Verification items for the finished model (mm, model axes). A direction names the side the tool comes from. Coordinates: 2 decimals unless noted, no trailing zeros. Order: outer loops, then holes, each group sorted by start corner. A loop starts at its lowest first (then second) coordinate and runs counter-clockwise, first axis right, second up. Notation, with made-up numbers: M 15.5,38 L 46.5,38 A27 ccw 46.5,70 Z; hole C -16,70.25 d7. An arc over 180 degrees is marked long. Return JSON: item names as keys, results as strings. Group by question number.
Q1. Thickness scan on probe 1 along X at (y, z) = (-2.75, 1); probe 2 along X at (y, z) = (6.75, 12); probe 3 along Y at (x, z) = (6.5, 3.5). Record the ranges inside material, lowest first.
Q2. Go/stop test with flat-tipped pins: pin 1 Ø3.5 at (x, z) = (5.64, -18.02) entering from +Y; pin 2 Ø1.8 at (x, y) = (0.64, 13) entering from +Z; pin 3 Ø6.5 at (x, z) = (0, -11.5) entering from -Y; pin 4 Ø6 at (x, z) = (5.5, 5.5) entering from +Y. Record where each tip stops, or that it passes through.
Q3. Section check C-C, the plane z = -17. Enter the section's corners in (x, y).
Q4. Section check A-A, the plane y = -4.25. Enter the section's corners in (x, z).
Q5. Section check B-B, the plane x = 0.75. Enter the section's corners in (y, z).
Q6. Section check D-D, the plane y = 3. Enter the section's corners in (x, z).
Q7. Access from +Z, -Z, +X, -X, +Y, -Y to the whole of each face (thin tool, end or side, straight path). Record for faces 5 (the face through (0, -3, 7)), 6 (the face through (0.318, 11.536, 16.512)), 7 (the face through (1, 8, 13.977)), 8 (the face through (-4, -1, -20.873)), 9 (the face through (-4.682, -3.972, -19.487)).
Q8. Mould release check, pull along Z, two halves, no side actions. Record for faces 1 (the face through (1, 0, -3)), 2 (the face through (-5.547, -3.972, 0.064)), 3 (the face through (-5.385, 8.112, 9.047)), 4 (the face through (7.976, -0.986, -16.363)): pulls with the +Z half, pulls with the -Z half, needs draft (parallel to the pull), parting line crosses it, or undercut.
from build123d import *

# Parameters (mm, degrees)
F0_W      = 16
F0_H      = 40
F0_R      = 1.5
F0_W_2    = 8
F0_H_2    = 14
F0_W_3    = 10
F0_H_3    = 4.5
F1_DEPTH  = 6
F2_DEPTH  = 3
F3_W      = 16
F3_H      = 16
F3_R      = 1.5
F4_DEPTH  = 5
F7_DEPTH  = 2
F9_DEPTH  = 4
F10_START = -12
F10_DEPTH = 4


with BuildPart() as f1:
    # F0 (on Front) → F1 (new body)
    with BuildSketch(Plane.XZ):
        with Locations((0.6433322058, -1.0231063997)):
            Rectangle(F0_W, F0_H)
        with Locations((-4.3566677942, -18.0231063997)):
            Circle(F0_R, mode=Mode.SUBTRACT)
        with Locations((0.6433322058, -8.5231063997)):
            Rectangle(F0_W_2, F0_H_2, mode=Mode.SUBTRACT)
        with Locations((5.6433322058, -18.0231063997)):
            Circle(F0_R, mode=Mode.SUBTRACT)
        with Locations((-4.3566677942, 0.9768936003)):
            Circle(F0_R, mode=Mode.SUBTRACT)
        with Locations((0.246625971, 7.2268936003)):
            Rectangle(F0_W_3, F0_H_3, mode=Mode.SUBTRACT)
        with Locations((5.6433322058, 0.9768936003)):
            Circle(F0_R, mode=Mode.SUBTRACT)
    extrude(amount=F1_DEPTH)

    # F0 (on Front) → F2 (join)
    with BuildSketch(Plane.XZ):
        with Locations((0.246625971, 7.2268936003)):
            Rectangle(F0_W_3, F0_H_3)
        with Locations((0.6433322058, -8.5231063997)):
            Rectangle(F0_W_2, F0_H_2)
    extrude(amount=F2_DEPTH)

    # F3 (on face) → F4 (join)
    with BuildSketch(Plane.XY.offset(18.9768936003)):
        with Locations((0.6433322058, 8)):
            Rectangle(F3_W, F3_H)
        with Locations((0.6433322058, 3)):
            Circle(F3_R, mode=Mode.SUBTRACT)
        with Locations((0.6433322058, 13)):
            Circle(F3_R, mode=Mode.SUBTRACT)
    extrude(amount=-F4_DEPTH)

    # F6 (on face) → F7 (cut)
    with BuildSketch(Plane.XZ):
        Polygon((7.288780473, 3.8268936003), (3.9978839386, 3.8268936003), (2.3524356714, 0.9768936003), (3.9978839386, -1.8731063997), (7.288780473, -1.8731063997), (8.9342287402, 0.9768936003), align=None)
        Polygon((-2.711219527, 3.8268936003), (-6.0021160614, 3.8268936003), (-7.6475643286, 0.9768936003), (-6.0021160614, -1.8731063997), (-2.711219527, -1.8731063997), (-1.0657712598, 0.9768936003), align=None)
        Polygon((-2.711219527, -15.1731063997), (-6.0021160614, -15.1731063997), (-7.6475643286, -18.0231063997), (-6.0021160614, -20.8731063997), (-2.711219527, -20.8731063997), (-1.0657712598, -18.0231063997), align=None)
        Polygon((7.288780473, -15.1731063997), (3.9978839386, -15.1731063997), (2.3524356714, -18.0231063997), (3.9978839386, -20.8731063997), (7.288780473, -20.8731063997), (8.9342287402, -18.0231063997), align=None)
    extrude(amount=F7_DEPTH, mode=Mode.SUBTRACT)

    # F8 (on face) → F9 (join)
    with BuildSketch(Plane(origin=(-7.3566677942, 0, 0), x_dir=(0, -1, 0), z_dir=(-1, 0, 0))):
        Polygon((-16, 13.9768936003), (0, 3.9768936003), (0, 13.9768936003), align=None)
    extrude(amount=-F9_DEPTH)

    # F8 (on face) → F10 (join)
    with BuildSketch(Plane(origin=(-7.3566677942, 0, 0), x_dir=(0, -1, 0), z_dir=(-1, 0, 0)).offset(F10_START)):
        Polygon((-16, 13.9768936003), (0, 3.9768936003), (0, 13.9768936003), align=None)
    extrude(amount=-F10_DEPTH)


solid = f1.part
Numbers:
{
 "1": {"probe 1": "x = -7.36 to -5.86, -2.86 to 4.14, 7.14 to 8.64", "probe 2": "x = -7.36 to -3.36, 4.64 to 8.64", "probe 3": "y = -6 to -2"},
 "2": {"pin 1": "stops at y = -2", "pin 2": "passes through", "pin 3": "stops at y = -3", "pin 4": "stops at y = 7.24"},
 "3": {"outline": "M -7.36,-6 L -5.45,-6 L -5.45,-2 L -7.06,-2 L -7.06,0 L -7.36,0 Z; M -3.26,-6 L 4.55,-6 L 4.55,-2 L 2.94,-2 L 2.94,0 L -1.66,0 L -1.66,-2 L -3.26,-2 Z; M 6.74,-6 L 8.64,-6 L 8.64,0 L 8.34,0 L 8.34,-2 L 6.74,-2 Z"},
 "4": {"outline": "M -7.36,-21.02 L 8.64,-21.02 L 8.64,18.98 L -7.36,18.98 Z; hole C -4.36,-18.02 d3; hole C -4.36,0.98 d3; hole M -4.75,4.98 L 5.25,4.98 L 5.25,9.48 L -4.75,9.48 Z; hole M -3.36,-15.52 L 4.64,-15.52 L 4.64,-1.52 L -3.36,-1.52 Z; hole C 5.64,-18.02 d3; hole C 5.64,0.98 d3"},
 "5": {"outline": "M -6,-21.02 L 0,-21.02 L 0,13.98 L 1.5,13.98 L 1.5,18.98 L -6,18.98 L -6,9.48 L -3,9.48 L -3,4.98 L -6,4.98 L -6,-1.52 L -3,-1.52 L -3,-15.52 L -6,-15.52 Z; M 4.5,13.98 L 11.5,13.98 L 11.5,18.98 L 4.5,18.98 Z; M 14.5,13.98 L 16,13.98 L 16,18.98 L 14.5,18.98 Z"},
 "6": {"outline": "M -7.36,5.85 L -3.36,5.85 L -3.36,13.98 L -0.86,13.98 L -0.86,18.98 L -7.36,18.98 Z; M 2.14,13.98 L 4.64,13.98 L 4.64,5.85 L 8.64,5.85 L 8.64,18.98 L 2.14,18.98 Z"},
 "7": {"face 5": "-Y", "face 6": "+Z, -Z", "face 7": "-Z, +Y", "face 8": "+Y", "face 9": "+Y, -Y"},
 "8": {"face 1": "needs draft", "face 2": "undercut", "face 3": "pulls with the -Z half", "face 4": "undercut"}
}
